Read the model definition and answer for the solid it produces. Units are mm, in the model's axes. Face numbers are marked on the shaded views. A direction names the side the tool comes from. Round coordinates to 2 decimals unless told otherwise and drop trailing zeros. Loops run counter-clockwise (first coordinate to the right, second up) from the corner with the lowest first, then second, coordinate; pieces in that order, holes last. Notation, with made-up numbers: M 69.5,38 L 74.5,38 A19 ccw 74.5,68 Z; hole C 38,65.25 d1. An arc over 180 degrees is marked long. Answer as CSV lines item,"result".
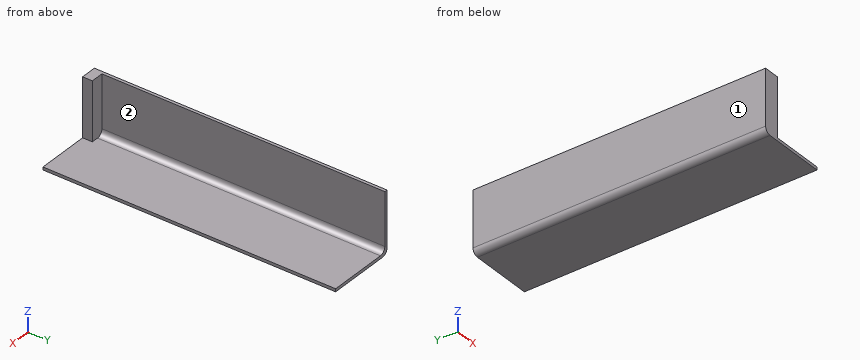
Autodesk Inventor part; units mm, degrees
ref_plane "YZ Plane" through (0, 0, 0) normal (1, 0, 0) x (0, 1, 0)
ref_plane "XZ Plane" through (0, 0, 0) normal (0, 1, 0) x (-1, 0, 0)
ref_plane "XY Plane" through (0, 0, 0) normal (0, 0, 1) x (1, 0, 0)
ref_plane "Arbeitsebene1" through (0, 0, 0) normal (0, 0, 1) x (1, 0, 0)
sketch "Skizze1" plane through (0, 0, 0) normal (0, 0, 1) x (1, 0, 0)
  line L0 (0, 0) -> (-35, 0)
  line L1 (-35, 0) -> (-35, -150)
  line L2 (-35, -150) -> (0, -150)
  line L3 (0, -150) -> (0, 0)
  dimension "d18" = 35
  dimension "d19" = 150
extrude "Extrusion1" add sketch "Skizze1" along normal blind 1.5
sketch "Skizze2" plane through (0, 0, 1.5) normal (0, 0, 1) x (1, 0, 0)
  line L0 (-35, 0) -> (-35, -150)
  line L1 (0, 0) -> (-35, 0)
  line L2 (0, -150) -> (0, 0)
  line L3 (-35, -150) -> (0, -150)
  line L4 (0, 0) -> (-35, 0)
  line L5 (-35, -150) -> (-33.5, -150)
  line L6 (-33.5, -150) -> (-33.5, 0)
  line L7 (-33.5, 0) -> (-35, 0)
  line L8 (-35, 0) -> (-35, -150)
  point P0 (0, -87)
  point P1 (-33.5, 0)
  dimension "d20" = 1.5
extrude "Extrusion2" add sketch "Skizze2" along normal blind 30 contours L1 L6 L3 L0
fillet "Rundung2" radius 3 2 edges at (-35, -75, 0) (-33.5, -75, 1.5)
sketch "Skizze6" plane through (-33.5, -150, 31.5) normal (1, 0, 0) x (0, 0, -1)
  line L0 (31.5, 0) -> (31.5, 150)
  line L1 (0, 0) -> (31.5, 0)
  line L2 (31.5, 0) -> (31.5, 5)
  line L3 (31.5, 5) -> (0, 5)
  line L4 (0, 5) -> (0, 0)
  line L5 (30.1312, 5) -> (30.1312, 0)
  dimension "d22" = 5
extrude "Extrusion6" add sketch "Skizze6" along normal blind 6.5 contours L1 L4 L3 L5
properties part number "50_Nema12_Linearmotor_150mm_cage"
1) Straight lines are drawn through the part: line 1 (X direction, y = -125, z = 24.5); line 2 (Y direction, x = -33, z = 9); line 3 (Z direction, x = -11, y = -14.5). For each, find the intervals that lie inside material, in ascending order.
Evaluation:
line 1,"x = -35 to -33.5"
line 2,"y = -150 to -145"
line 3,"z = 0 to 1.5"
2) Find section C-C, the plane x = -4. Give the vertices of the cut face in (y, z).
Evaluation:
outline,"M -150,0 L 0,0 L 0,1.5 L -150,1.5 Z"
3) Find section B-B, the plane z = 20.5. Give the vertices of the cut face in (x, y), then the cut area to 4 significant figures.
Evaluation:
outline,"M -35,-150 L -27,-150 L -27,-145 L -33.5,-145 L -33.5,0 L -35,0 Z"
area,"257.5 mm^2"
4) Each of these flat-tipped pins is pushed along its axis until it touches: P1, Ø8, axis at y = -107, z = 15, coming from the +X side; P2, Ø2.5, axis at y = -148, z = 16.5, coming from the +X side; P3, Ø5, axis at x = -22.5, y = -125.5, coming from the +Z side; P4, Ø8, axis at x = -20, z = 26, coming from the -Y side. Where does it stop, or does it pass through?
Evaluation:
P1,"stops at x = -33.5"
P2,"stops at x = -27"
P3,"stops at z = 1.5"
P4,"passes through"
5) Find section A-A, the plane y = -117.5. Give the vertices of the cut face in (x, z).
Evaluation:
outline,"M -35,3 A3 ccw -32,0 L 0,0 L 0,1.5 L -30.5,1.5 A3 cw -33.5,4.5 L -33.5,31.5 L -35,31.5 Z"
6) A tool of negligible diameter and unlimited length cuts with its end or side. For the marked faces 1 and 2, from which of +Z, -Z, +X, -X, +Y, -Y can it reach the whole face along a straight path? Write none if from no direction.
Evaluation:
face 1,"+Z, -Z, -X, +Y, -Y"
face 2,"+Z, +X, +Y"
